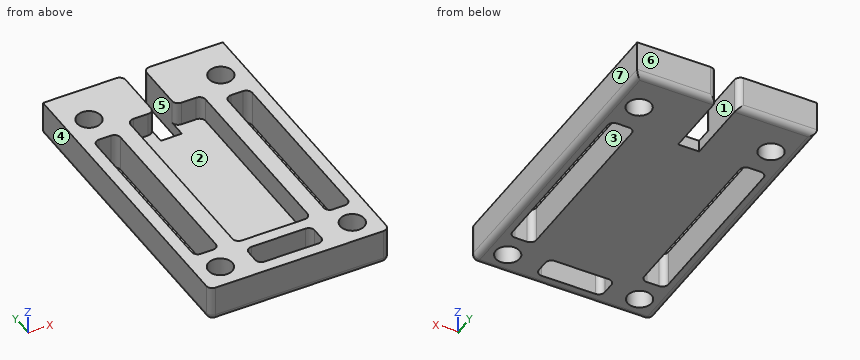
Solid Edge part; units mm, degrees
sketch "Sketch1" plane through (0, 0, 0) normal (0, 0, 1) x (1, 0, 0)
  line L0 (-15, -25.345) -> (15, -25.345)
  line L1 (15, -25.345) -> (15, 25.345)
  line L2 (15, 25.345) -> (-15, 25.345)
  line L3 (-15, 25.345) -> (-15, -25.345)
  dimension "D1" = 15
  dimension "D2" = 15
extrude "Protrusion1" add sketch "Sketch1" along normal blind 6
hole "Hole1" at (-11, 18.655, 6) direction (0, 0, -1) diameter 4 end up to next
hole "Hole2" at (11, 18.655, 6) direction (0, 0, -1) diameter 4 end up to next
hole "Hole3" at (-11, -21.345, 6) direction (0, 0, -1) diameter 4 end up to next
hole "Hole4" at (11, -21.345, 6) direction (0, 0, -1) diameter 4 end up to next
sketch "Sketch2" plane through (0, 0, 0) normal (0, 0, -1) x (1, 0, 0)
  line L0 (1.76, -25.345) -> (-1.76, -25.345)
  line L1 (-1.76, -25.345) -> (-1.76, -13.655)
  line L2 (-1.76, -13.655) -> (1.76, -13.655)
  line L3 (1.76, -13.655) -> (1.76, -25.345)
  dimension "D1" = 1.76
  dimension "D2" = 1.76
extrude "Cutout1" cut sketch "Sketch2" against normal through all
sketch "Sketch3" plane through (0, 0, 6) normal (0, 0, 1) x (0, 1, 0)
  line L0 (-17.345, -6.25) -> (15.655, -6.25)
  line L1 (15.655, -6.25) -> (15.655, 6.25)
  line L2 (15.655, 6.25) -> (-17.345, 6.25)
  line L3 (-17.345, 6.25) -> (-17.345, -6.25)
  dimension "D1" = 17.345
  dimension "D2" = 17.345
extrude "Utskärning_för_batteriet" cut sketch "Sketch3" against normal blind 4
sketch "Sketch4" plane through (0, 0, 6) normal (0, 0, 1) x (-1, 0, 0)
  line L0 (-5.26, 23.345) -> (5.74, 23.345)
  line L1 (5.74, 23.345) -> (5.74, 19.345)
  line L2 (5.74, 19.345) -> (-5.26, 19.345)
  line L3 (-5.26, 19.345) -> (-5.26, 23.345)
  line L4 (9, 17.265) -> (13, 17.265)
  line L5 (13, 17.265) -> (13, -13.735)
  line L6 (13, -13.735) -> (9, -13.735)
  line L7 (9, -13.735) -> (9, 17.265)
  line L8 (-13, 17.265) -> (-9, 17.265)
  line L9 (-9, 17.265) -> (-9, -13.735)
  line L10 (-9, -13.735) -> (-13, -13.735)
  line L11 (-13, -13.735) -> (-13, 17.265)
  dimension "D1" = 5.26
  dimension "D2" = 5.26
extrude "Cutout2" cut sketch "Sketch4" against normal through all
fillet "Avrundningar_1" radius 1 27 edges at (-15, 0, 0) (0, -25.345, 0) (15, 0, 0) (-15, -25.345, 3) (15, -25.345, 3) (-8.38, 25.345, 0) (-1.76, 25.345, 3) (1.76, 25.345, 3) (8.38, 25.345, 0) (6.25, -17.345, 4) (-6.25, -17.345, 4) (-6.25, 15.655, 4) (6.25, 15.655, 4) (13, -17.265, 3) (9, -17.265, 3) (9, 13.735, 3) (13, 13.735, 3) (-9, 13.735, 3) (-13, 13.735, 3) (-13, -17.265, 3) (-9, -17.265, 3) (5.26, -23.345, 3) (-5.74, -23.345, 3) (5.26, -19.345, 3) (-5.74, -19.345, 3) (1.76, 15.655, 4) (-1.76, 15.655, 4)
The model under review builds one solid part; all positions refer to its coordinate system, in mm. Face numbers are marked on the shaded views. A direction names the side the tool comes from. Round coordinates to 2 decimals unless told otherwise and drop trailing zeros. Loops run counter-clockwise (first coordinate to the right, second up) from the corner with the lowest first, then second, coordinate; pieces in that order, holes last. Notation, with made-up numbers: M 1,-20.75 L 52,-20.75 A22 cw 52,18.25 Z; hole C 76.5,9.25 d8. An arc over 180 degrees is marked long. Answer as CSV lines item,"result". Start each with the question number.
Item 1: Consider section A-A (x = 11). Write out the cut boundary in (y, z) (3 decimals).
Item 2: Consider section D-D (z = 4.75). State how many separate pieces and enclosed holes the cut face has, then the cut area to 3 significant figures.
Item 3: Consider section C-C (y = -8.5). Write out the cut boundary in (x, z), then the cut area to 3 significant figures.
Item 4: Wall thickness on line 1 (X direction, y = -8, z = 5); line 2 (Y direction, x = 11, z = 2.75) (3 decimals); line 3 (Y direction, x = -1.5, z = 3.75) (3 decimals): over which ranges is each line inside the solid? List them lowest first. Write a range as [from, to].
Item 5: For the marked faces 1, 2 and 3, list the 3-axis set-ups (+Z, -Z, +X, -X, +Y, -Y) from which the entire face can be reached by the end or side of a thin tool; tool diameter is ignored.
Item 6: Mouldability with a two-part tool opening along X and no side actions: class the marked faces 4, 5, 6 and 7 as released by +X, released by -X, zero draft, split by the parting line, or undercut.
Item 7: Consider section B-B (y = 22.5). Write out the cut boundary in (x, z), then the cut area to 3 significant figures.
Item 8: Insertion check: P1, Ø5, axis at x = -0.5, y = 5, coming from the -Z side; P2, Ø2, axis at x = -0.5, z = 1, coming from the +Y side (3 decimals). Each pin has a flat end and moves straight along its axis. Give the tip position at first contact, or say it passes through.
Answer:
1,outline,"M -25.345,1 A1 ccw -24.345,0 L -23.345,0 L -23.345,6 L -25.345,6 Z; M -19.345,0 L -17.265,0 L -17.265,6 L -19.345,6 Z; M 13.735,0 L 16.655,0 L 16.655,6 L 13.735,6 Z; M 20.655,0 L 24.345,0 A1 ccw 25.345,1 L 25.345,6 L 20.655,6 Z"
2,separate pieces,"1"
2,enclosed holes,"7"
2,area,"734 mm^2"
3,outline,"M -15,1 A1 ccw -14,0 L -13,0 L -13,6 L -15,6 Z; M -9,0 L 9,0 L 9,6 L 6.25,6 L 6.25,2 L -6.25,2 L -6.25,6 L -9,6 Z; M 13,0 L 14,0 A1 ccw 15,1 L 15,6 L 13,6 Z"
3,area,"81.6 mm^2"
4,line 1,"x = [-15, -13], [-9, -6.25], [6.25, 9], [13, 15]"
4,line 2,"y = [-25.345, -23.345], [-19.345, -17.265], [13.735, 16.655], [20.655, 25.345]"
4,line 3,"y = [-25.345, -23.345], [-19.345, -17.345]"
5,face 1,"+Z, -Z, +Y"
5,face 2,"+Z"
5,face 3,"+Z, -Z"
6,face 4,"released by -X"
6,face 5,"undercut"
6,face 6,"zero draft"
6,face 7,"released by +X"
7,outline,"M -15,1 A1 ccw -14,0 L -1.76,0 L -1.76,6 L -15,6 Z; M 1.76,0 L 14,0 A1 ccw 15,1 L 15,6 L 1.76,6 Z"
7,area,"158 mm^2"
8,P1,"stops at z = 0"
8,P2,"stops at y = 13.655"
